from build123d import *

# Parameters (mm, degrees)
SKETCH1_W           = 62.4
SKETCH1_H           = 22.5
BOSS_EXTRUDE1_DEPTH = 18.8
SKETCH2_R           = 1.8
BOSS_EXTRUDE2_DEPTH = 9.8
BOSS_EXTRUDE3_START = 9.8
SKETCH3_R           = 1.8
BOSS_EXTRUDE3_DEPTH = 9.8


with BuildPart() as part:
    # Sketch1 → Boss-Extrude1 (new body)
    with BuildSketch(Plane.XY):
        Rectangle(SKETCH1_W, SKETCH1_H)
    extrude(amount=BOSS_EXTRUDE1_DEPTH)

    # Sketch2 → Boss-Extrude2 (add)
    with BuildSketch(Plane.XY.offset(18.8)):
        with Locations((-20, 0)):
            Circle(SKETCH2_R)
    extrude(amount=BOSS_EXTRUDE2_DEPTH)

    # Sketch3 → Boss-Extrude3 (add)
    with BuildSketch(Plane(origin=(0, 0, 0), x_dir=(-1, 0, 0), z_dir=(0, 0, -1)).offset(BOSS_EXTRUDE3_START)):
        with Locations(Location((20, 0, 0), (0, 0, 180))):
            Circle(SKETCH3_R)
    extrude(amount=-BOSS_EXTRUDE3_DEPTH)


solid = part.part
Could you check a few things on this model? Use its own coordinates, in mm. A direction names the side the tool comes from. Give positions to 0.01 mm unless a question says otherwise; leave off trailing zeros. Order: outer loops, then holes, each group sorted by start corner. A loop starts at its lowest first (then second) coordinate and runs counter-clockwise, first axis right, second up. Notation, with made-up numbers: (57.5, -40) -> (61.5, -40) arc R22 ccw to (61.5, -11) -> close; hole circle Ø5 at (-13, 38.25). An arc over 180 degrees is marked (long way). Return JSON: item names as keys, results as strings.
1. Imagine slicing it at C-C on z = -1. List the corners of the cut face in (x, y) for me, then the cut area to 3 significant figures.
Answer list:
{"outline": "circle Ø3.6 at (-20, 0)", "area": "10.2 mm2"}
2. I need wall thicknesses on line 1 (Z direction, x = -2.5, y = -0.75). Which ranges of the line are inside material? Lowest first, please. Write a range as from..to.
Answer list:
{"line 1": "z = 0..18.8"}
3. Imagine slicing it at A-A on y = 0. List the corners of the cut face in (x, z) for me, then the cut area to 3 significant figures.
Answer list:
{"outline": "(-31.2, 0) -> (-21.8, 0) -> (-21.8, -9.8) -> (-18.2, -9.8) -> (-18.2, 0) -> (31.2, 0) -> (31.2, 18.8) -> (-18.2, 18.8) -> (-18.2, 28.6) -> (-21.8, 28.6) -> (-21.8, 18.8) -> (-31.2, 18.8) -> close", "area": "1,240 mm2"}
4. Imagine slicing it at D-D on y = 8.5. List the corners of the cut face in (x, z) for me.
Answer list:
{"outline": "(-31.2, 0) -> (31.2, 0) -> (31.2, 18.8) -> (-31.2, 18.8) -> close"}
5. Imagine slicing it at B-B on x = -20. List the corners of the cut face in (y, z) for me.
Answer list:
{"outline": "(-11.25, 0) -> (-1.8, 0) -> (-1.8, -9.8) -> (1.8, -9.8) -> (1.8, 0) -> (11.25, 0) -> (11.25, 18.8) -> (1.8, 18.8) -> (1.8, 28.6) -> (-1.8, 28.6) -> (-1.8, 18.8) -> (-11.25, 18.8) -> close"}
6. On a 3-axis mill with a long thin cutter (end or side, diameter ignored), from which of +Z, -Z, +X, -X, +Y, -Y can I reach the whole of each face in a straight line? I mean faces 1 (the cylindrical face through (-18.283, 0.541, 23.631)), 2 (the flat face through (-20, 0, 28.6)), 3 (the cylindrical face through (-18.283, -0.541, -4.969)). Say none if no direction works.
Answer list:
{"face 1": "+Z", "face 2": "+Z, +X, -X, +Y, -Y", "face 3": "-Z"}
7. For pin 1 Ø2 at (x, y) = (2.5, 3) entering from +Z; pin 2 Ø1.5 at (x, y) = (7, -8) entering from -Z; pin 3 Ø2 at (y, z) = (-0.5, -1.5) entering from +X, each with a flat end and sliding along its axis, tell me the tip position at first contact or that it passes through.
Answer list:
{"pin 1": "stops at z = 18.8", "pin 2": "stops at z = 0", "pin 3": "stops at x = -18.2"}
